Model file for the job. Use its own axes, mm. A direction names the side the tool comes from. Coordinates: 2 decimals unless noted, no trailing zeros. Write each loop counter-clockwise with the first axis right and the second up, starting at its lowest first coordinate (ties: lowest second). Pieces come first, ordered by that corner, then holes.
Q1. Which spindle directions (+Z, -Z, +X, -X, +Y, -Y) get a long thin tool onto all of the face, cutting with end or side? Do faces 1 (the flat face through (900, 10, 1)), 2 (the flat face through (849, -10, -1)), 3 (the flat face through (-849, -10, -1)). Say none if no direction does.
Q2. Drill centre line: probe 1 along X at (y, z) = (-19.5, -9). Where is it in solid material? Low to high.
Q3. Band-saw the part on A-A, the plane z = -33. Write the cut outline in (x, y).
from build123d import *

# Parameters (mm, degrees)
F1_W     = 60
F1_H     = 100
F2_DEPTH = 800
F3_W     = 40
F3_H     = 100
F4_DEPTH = 100


# Not quite as in the source:
# - a pattern or mirror of a feature is missing from the dataset's text; its kind, count and spacing are read off the source's solid


with BuildPart() as f2:
    # F1 (on Right) → F2 (new body, symmetric)
    with BuildSketch(Plane.YZ):
        Rectangle(F1_W, F1_H)
    extrude(amount=F2_DEPTH, both=True)

    # F3 (on face) → F4 (join)
    with BuildSketch(Plane(origin=(-800, 0, 0), x_dir=(0, -1, 0), z_dir=(-1, 0, 0))):
        with Locations((-10, 0)):
            Rectangle(F3_W, F3_H)
    f4 = extrude(amount=F4_DEPTH)

    # F4_copies: F4 across plane
    add(f4.mirror(Plane(origin=(0, 0, 0), x_dir=(0, 0, 1), z_dir=(1, 0, 0))))


solid = f2.part
Answer sheet:
1. face 1: +Z, -Z, +X, +Y, -Y
1. face 2: +Z, -Z, +X, -Y
1. face 3: +Z, -Z, -X, -Y
2. probe 1: x = -800 to 800
3. outline: (-900, -10) - (-800, -10) - (-800, -30) - (800, -30) - (800, -10) - (900, -10) - (900, 30) - (-900, 30) - close
